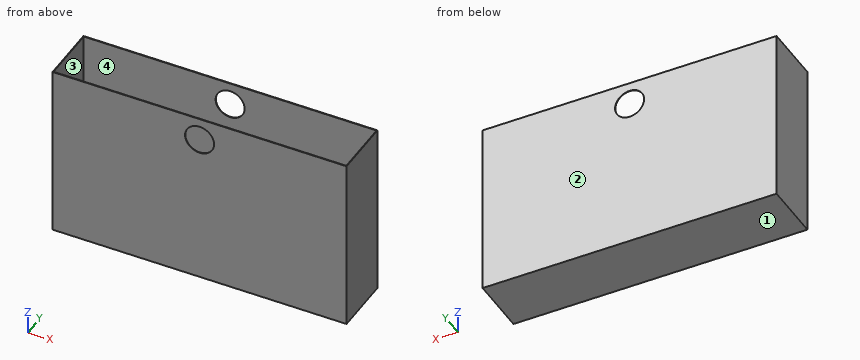
```python
from build123d import *

# Parameters (mm, degrees)
F0_W     = 127
F0_H     = 76.2
F1_DEPTH = 25.4
F2_T     = -0.254
F3_R     = 6.272881
F4_DEPTH = 50.8


with BuildPart() as f1:
    # F0 (on Front) → F1 (new body)
    with BuildSketch(Plane.XZ):
        Rectangle(F0_W, F0_H)
    extrude(amount=F1_DEPTH)

    # F2
    f2_openings = [f1.faces().sort_by_distance(p)[0] for p in [
        (0, -12.7, 38.1),
    ]]
    offset(amount=F2_T, openings=f2_openings)

    # F3 (on face) → F4 (cut)
    with BuildSketch(Plane.XZ.offset(25.4)):
        with Locations((0, 28.13966)):
            Circle(F3_R)
    extrude(amount=-F4_DEPTH, mode=Mode.SUBTRACT)


solid = f1.part
```
Work out the finished part from the listing and answer in its coordinate system (mm). Face numbers are marked on the shaded views. Round coordinates to 2 decimals unless told otherwise and drop trailing zeros. Loops run counter-clockwise (first coordinate to the right, second up) from the corner with the lowest first, then second, coordinate; pieces in that order, holes last.
(1) The part is cut by section C-C, the plane y = -4.5. Give the vertices of the cut face in (x, z).
Computed values:
outline: (-63.5, -38.1) - (63.5, -38.1) - (63.5, 38.1) - (63.25, 38.1) - (63.25, -37.85) - (-63.25, -37.85) - (-63.25, 38.1) - (-63.5, 38.1) - close
(2) Find the intervals of material crossed by L1, parallel to X at y = -14.5, z = 34.5; L2, parallel to Z at x = 0, y = -25.25; L3, parallel to Y at x = -45.5, z = -30, in increasing order.
Computed values:
L1: x = -63.5 to -63.25, 63.25 to 63.5
L2: z = -38.1 to 21.87, 34.41 to 38.1
L3: y = -25.4 to -25.15, -0.25 to 0
(3) The part is cut by section D-D, the plane x = -43. Give the vertices of the cut face in (y, z).
Computed values:
outline: (-25.4, -38.1) - (0, -38.1) - (0, 38.1) - (-0.25, 38.1) - (-0.25, -37.85) - (-25.15, -37.85) - (-25.15, 38.1) - (-25.4, 38.1) - close
(4) The mould has two halves that part along Y. Classify the marked faces 1, 2, 3 and 4: pulls with the +Y half, pulls with the -Y half, needs draft (parallel to the pull), parting line crosses it, or undercut.
Computed values:
face 1: needs draft
face 2: pulls with the +Y half
face 3: undercut
face 4: undercut
(5) The part is cut by section B-B, the plane z = 17.5. Give the vertices of the cut face in (x, y).
Computed values:
outline: (-63.5, -25.4) - (63.5, -25.4) - (63.5, 0) - (-63.5, 0) - close; hole (-63.25, -25.15) - (63.25, -25.15) - (63.25, -0.25) - (-63.25, -0.25) - close
(6) The part is cut by section A-A, the plane x = 1. Give the vertices of the cut face in (y, z), and give its area (3 significant figures).
Computed values:
outline: (-25.4, -38.1) - (0, -38.1) - (0, 21.95) - (-0.25, 21.95) - (-0.25, -37.85) - (-25.15, -37.85) - (-25.15, 21.95) - (-25.4, 21.95) - close; (-25.4, 34.33) - (-25.15, 34.33) - (-25.15, 38.1) - (-25.4, 38.1) - close; (-0.25, 34.33) - (0, 34.33) - (0, 38.1) - (-0.25, 38.1) - close
area: 38.7 mm2
(7) This flat-tipped pin is pushed along its axis until it touches: P1, Ø7.5, axis at x = -26.5, y = -14, coming from the +Z side. Where does it stop, or does it pass through?
Computed values:
P1: stops at z = -37.85
